from build123d import *

# Parameters (mm, degrees)
CROQUIS1_W              = 14
CROQUIS1_H              = 25
SALIENTE_EXTRUIR3_DEPTH = 21
CROQUIS3_W              = 14
CROQUIS3_H              = 25
SALIENTE_EXTRUIR4_DEPTH = 2
SALIENTE_EXTRUIR5_DEPTH = 3


with BuildPart() as part:
    # Croquis1 → Saliente-Extruir3 (new body)
    with BuildSketch(Plane.XY):
        Polygon((-26.265270251, -2.501993068), (-26.265270251, -29.501993068), (-10.265270251, -29.501993068), (-8.265270251, -29.501993068), (-8.265270251, -27.501993068), (-8.265270251, -0.501993068), (-24.265270251, -0.501993068), (-26.265270251, -0.501993068), align=None)
        with Locations((-17.265270251, -15.001993068)):
            Rectangle(CROQUIS1_W, CROQUIS1_H, mode=Mode.SUBTRACT)
    extrude(amount=SALIENTE_EXTRUIR3_DEPTH)

    # Croquis3 → Saliente-Extruir4 (add)
    with BuildSketch(Plane.XY.offset(21)):
        with Locations((-17.265270251, -15.001993068)):
            Rectangle(CROQUIS3_W, CROQUIS3_H)
    extrude(amount=-SALIENTE_EXTRUIR4_DEPTH)

    # Croquis4 → Saliente-Extruir5 (add)
    with BuildSketch(Plane.XY.offset(21)):
        Polygon((-56.265270251, 29.498006932), (-52.729736345, 33.033540838), (-19.194202439, -0.501993068), (-26.265270251, -0.501993068), (-26.265270251, -7.573060879), (-59.800804157, 25.962473026), align=None)
        Polygon((21.734729749, 29.498006932), (25.270263655, 25.962473026), (-8.265270251, -7.573060879), (-8.265270251, -0.501993068), (-15.336338063, -0.501993068), (18.199195843, 33.033540838), align=None)
        Polygon((25.270263655, -55.966459162), (21.734729749, -59.501993068), (18.199195843, -63.037526974), (-15.336338063, -29.501993068), (-8.265270251, -29.501993068), (-8.265270251, -22.430925256), align=None)
        Polygon((-56.265270251, -59.501993068), (-59.800804157, -55.966459162), (-26.265270251, -22.430925256), (-26.265270251, -29.501993068), (-19.194202439, -29.501993068), (-52.729736345, -63.037526974), align=None)
    extrude(amount=-SALIENTE_EXTRUIR5_DEPTH)


solid = part.part
Geometry: final body of the model. Coordinates: model frame, mm. A direction names the side the tool comes from. Give positions to 0.01 mm unless a question says otherwise; leave off trailing zeros. Write each loop counter-clockwise with the first axis right and the second up, starting at its lowest first coordinate (ties: lowest second). Pieces come first, ordered by that corner, then holes. Notation, with made-up numbers: (-1, 35) -> (9, 35) arc R26 cw to (9, 57) -> close; hole circle Ø10 at (-9, 14.5). An arc over 180 degrees is marked (long way). Answer as a JSON object with one key per item and string values.
1. Ray query, probe 1 along Y at (x, z) = (-21, 4.25); probe 2 along X at (y, z) = (-4, 9.5); probe 3 along Y at (x, z) = (-54, 19.25). Return the intervals inside material, ascending. Write a range as from..to.
Ans:
{"probe 1": "y = -29.5..-27.5, -2.5..-0.5", "probe 2": "x = -26.27..-24.27, -10.27..-8.27", "probe 3": "y = -61.77..-50.17, 20.16..31.76"}
2. Cut plane A-A on z = 2.75. Output: boundary loops of the cut face in (x, y), and give its area (3 significant figures).
Ans:
{"outline": "(-26.27, -29.5) -> (-8.27, -29.5) -> (-8.27, -0.5) -> (-26.27, -0.5) -> close; hole (-24.27, -27.5) -> (-10.27, -27.5) -> (-10.27, -2.5) -> (-24.27, -2.5) -> close", "area": "172 mm^2"}
3. Mould query, pull axis Y, two halves, no side actions, for faces 4 (the flat face through (21.685, -59.551, 19.521)), 5 (the flat face through (8.74, 9.43, 19.52)), 6 (the flat face through (-36.197, 16.501, 19.521)). Classes: pulls with the +Y half, pulls with the -Y half, needs draft (parallel to the pull), parting line crosses it, or undercut.
Ans:
{"face 4": "pulls with the -Y half", "face 5": "undercut", "face 6": "pulls with the +Y half"}
4. Cut plane B-B on x = -42. Output: boundary loops of the cut face in (y, z), and give its area (3 significant figures).
Ans:
{"outline": "(-52.31, 18) -> (-38.17, 18) -> (-38.17, 21) -> (-52.31, 21) -> close; (8.16, 18) -> (22.3, 18) -> (22.3, 21) -> (8.16, 21) -> close", "area": "84.9 mm^2"}
5. Cut plane C-C on y = 4. Output: boundary loops of the cut face in (x, z), and give its area (3 significant figures).
Ans:
{"outline": "(-37.84, 18) -> (-23.7, 18) -> (-23.7, 21) -> (-37.84, 21) -> close; (-10.83, 18) -> (3.31, 18) -> (3.31, 21) -> (-10.83, 21) -> close", "area": "84.9 mm^2"}
6. Contact query for flat-ended pins moving along their axis: pin 1 (1.5 mm diameter, centred on x = -23.5, z = 12, fed in from -Y); pin 2 (6 mm diameter, centred on y = -37, z = 18, fed in from +X); pin 3 (4 mm diameter, centred on x = -19.5, y = -15, fed in from -Z). Output: stop coordinate, or through.
Ans:
{"pin 1": "stops at y = -29.5", "pin 2": "stops at x = 9.3", "pin 3": "stops at z = 19"}
7. Cut plane D-D on y = -10. Output: boundary loops of the cut face in (x, z), and give its area (3 significant figures).
Ans:
{"outline": "(-26.27, 0) -> (-24.27, 0) -> (-24.27, 19) -> (-10.27, 19) -> (-10.27, 0) -> (-8.27, 0) -> (-8.27, 21) -> (-26.27, 21) -> close", "area": "112 mm^2"}
8. Access query for faces 1 (the flat face through (8.268, -38.964, 19.521)), 2 (the flat face through (-35.73, -46.04, 19.52)), 3 (the flat face through (-17, -15, 19)). Directions: +Z, -Z, +X, -X, +Y, -Y. A direction counts if a zero-diameter tool reaches every point of the face in a straight line with its end or side. Return the directions, or none.
Ans:
{"face 1": "+Z, -Z, +X", "face 2": "+Z, -Z, -Y", "face 3": "-Z"}
